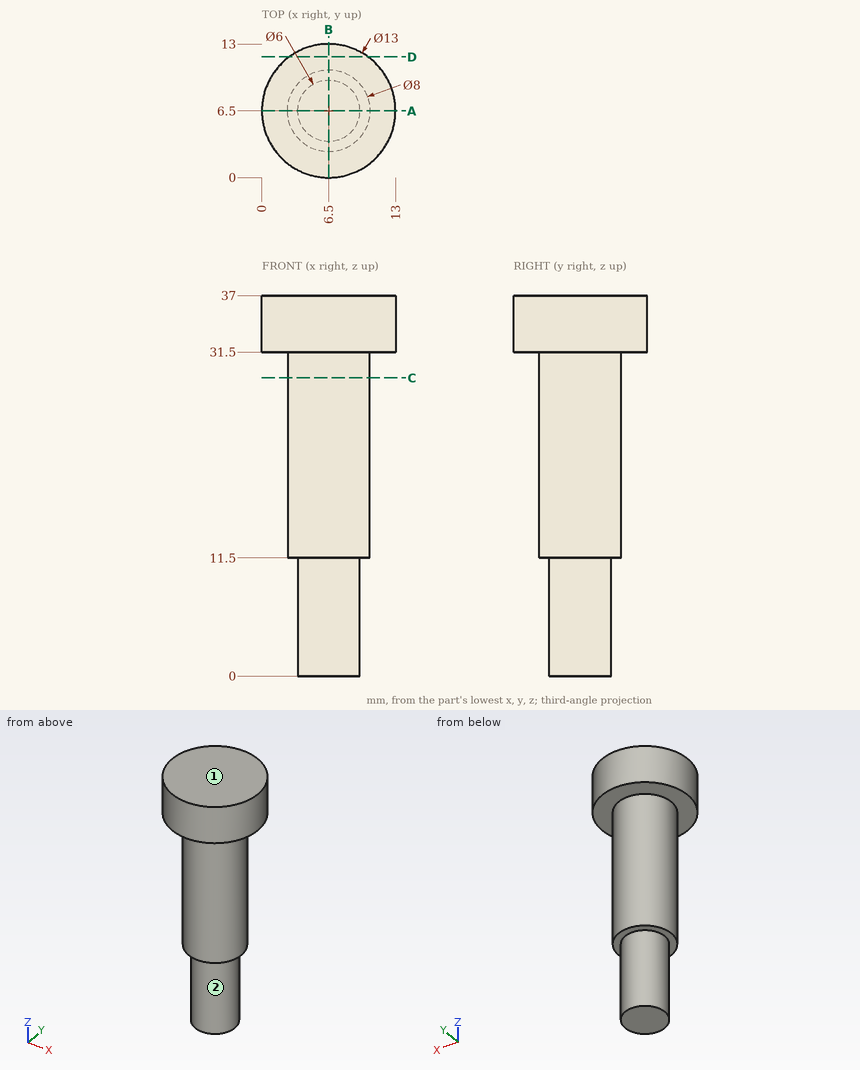
Can you work these out from the drawing? Everything is in mm from the part's minimum corner. A direction names the side the tool comes from. Coordinates: 2 decimals unless noted, no trailing zeros. Loops run counter-clockwise (first coordinate to the right, second up) from the corner with the lowest first, then second, coordinate; pieces in that order, holes last.
1. Imagine slicing it at A-A, the plane y = 6.5. Please give me the cut outline in (x, z), and give its area (4 significant figures).
2. I need wall thicknesses on L1, parallel to Z at x = 7.25, y = 3; L2, parallel to Z at x = 2.75, y = 5; L3, parallel to X at y = 12.25, z = 34.5. Which ranges of each line are inside material? Lowest first, please.
3. Imagine slicing it at C-C, the plane z = 29. Please give me the cut outline in (x, y).
4. Imagine slicing it at D-D, the plane y = 11.75. Please give me the cut outline in (x, z), and give its area (3 significant figures).
5. For P1, Ø6, axis at y = 8, z = 21, coming from the +X side; P2, Ø3, axis at x = 2.5, z = 21.5, coming from the +Y side; P3, Ø1, axis at x = 5.5, z = 27.5, coming from the -Y side, each with a flat end and sliding along its axis, tell me the tip position at first contact or that it passes through.
6. For the marked faces 1 and 2, which set-ups out of +Z, -Z, +X, -X, +Y, -Y let a thin tool reach every point of the face, with its end or its side?
Taken from the geometry:
1. outline: (0, 31.5) - (2.5, 31.5) - (2.5, 11.5) - (3.5, 11.5) - (3.5, 0) - (9.5, 0) - (9.5, 11.5) - (10.5, 11.5) - (10.5, 31.5) - (13, 31.5) - (13, 37) - (0, 37) - close
1. area: 300.5 mm2
2. L1: z = 11.5 to 37
2. L2: z = 31.5 to 37
2. L3: x = 3.47 to 9.53
3. outline: circle Ø8 at (6.5, 6.5)
4. outline: (2.67, 31.5) - (10.33, 31.5) - (10.33, 37) - (2.67, 37) - close
4. area: 42.2 mm2
5. P1: stops at x = 10.5
5. P2: stops at y = 9.62
5. P3: stops at y = 2.53
6. face 1: +Z, +X, -X, +Y, -Y
6. face 2: -Z
